Here's the drawing with two shaded views (mm, measured from the low corner). I have some questions. A direction names the side the tool comes from. Give positions to 0.01 mm unless a question says otherwise; leave off trailing zeros. Write each loop counter-clockwise with the first axis right and the second up, starting at its lowest first coordinate (ties: lowest second). Pieces come first, ordered by that corner, then holes. Notation, with made-up numbers: (59.5, 77.5) -> (77.5, 77.5) arc R20 cw to (77.5, 99.5) -> close; hole circle Ø4 at (84.25, 12.5). An arc over 180 degrees is marked (long way). One line per question, with ' | ' between items.
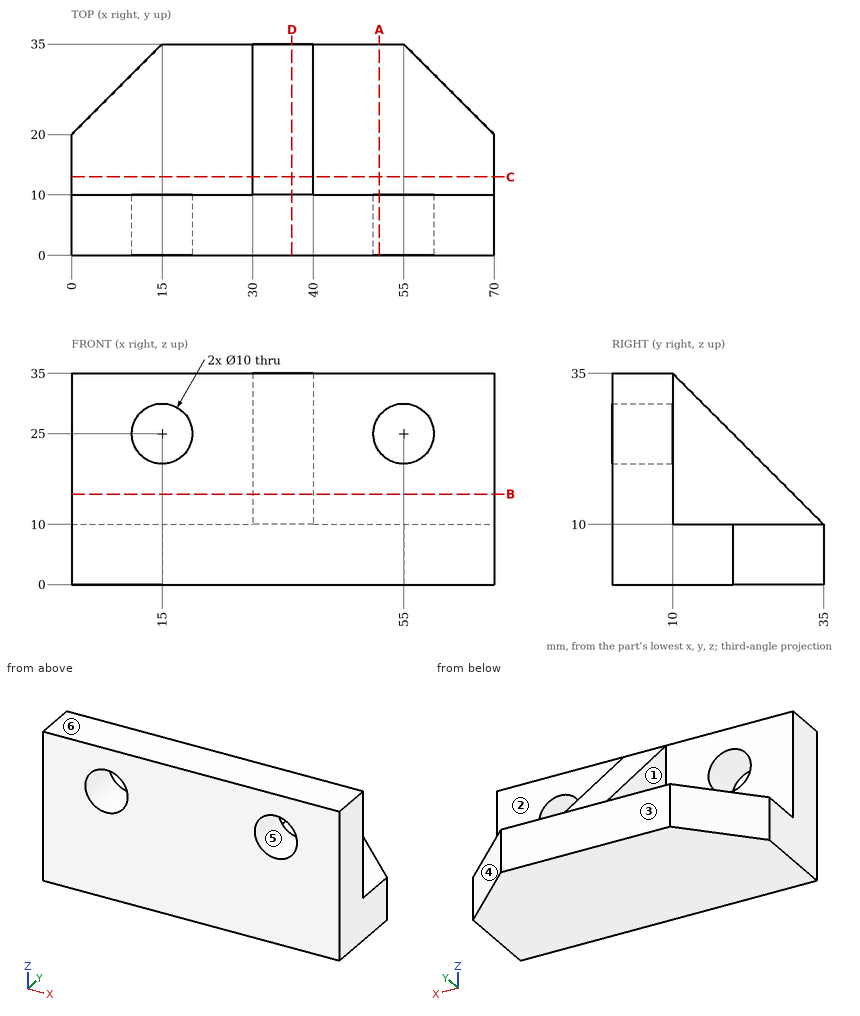
Q1. If we mould it in two halves opening along Z, with no side actions, what happens to the marked faces 4, 5 and 6? For each: +Z half, -Z half, draft (parallel to the pull), parting line (faces both ways), or undercut.
Answer below:
face 4: draft | face 5: undercut | face 6: +Z half
Q2. On a 3-axis mill with a long thin cutter (end or side, diameter ignored), from which of +Z, -Z, +X, -X, +Y, -Y can I reach the whole of each face in a straight line? I mean the marked faces 1, 2 and 3. Say none if no direction works.
Answer below:
face 1: +Z, -X, +Y | face 2: +Z, +X, +Y | face 3: +Z, -Z, +X, -X, +Y
Q3. Imagine slicing it at A-A on x = 51. Please give me the cut outline in (y, z).
Answer below:
outline: (0, 0) -> (35, 0) -> (35, 10) -> (10, 10) -> (10, 22) -> (0, 22) -> close; (0, 28) -> (10, 28) -> (10, 35) -> (0, 35) -> close
Q4. If I drill on line 1 along X through (y, z) = (2, 25); line 2 along Z through (x, y) = (15, 6.75); line 3 along Y through (x, z) = (48.5, 14), over which ranges is the centre line in solid material (lowest first)?
Answer below:
line 1: x = 0 to 10, 20 to 50, 60 to 70 | line 2: z = 0 to 20, 30 to 35 | line 3: y = 0 to 10
Q5. Imagine slicing it at C-C on y = 13. Please give me the cut outline in (x, z).
Answer below:
outline: (0, 0) -> (70, 0) -> (70, 10) -> (40, 10) -> (40, 32) -> (30, 32) -> (30, 10) -> (0, 10) -> close
Q6. Imagine slicing it at D-D on x = 36.5. Please give me the cut outline in (y, z).
Answer below:
outline: (0, 0) -> (35, 0) -> (35, 10) -> (10, 35) -> (0, 35) -> close
Q7. Imagine slicing it at B-B on z = 15. Please give me the cut outline in (x, y).
Answer below:
outline: (0, 0) -> (70, 0) -> (70, 10) -> (40, 10) -> (40, 30) -> (30, 30) -> (30, 10) -> (0, 10) -> close
Q8. Will these pins go through, and if not, where does the flat tip stop? pin 1 (6 mm diameter, centred on y = 28.5, z = 7.5, fed in from -X); pin 2 (12 mm diameter, centred on x = 32.5, y = 28, fed in from +Z); pin 3 (9 mm diameter, centred on x = 55, z = 25, fed in from +Y); pin 4 (6 mm diameter, centred on y = 16.5, z = 16.5, fed in from -X).
Answer below:
pin 1: stops at x = 5.5 | pin 2: stops at z = 23 | pin 3: passes through | pin 4: stops at x = 30
